Part model, mm, in its own coordinate system. A direction names the side the tool comes from. Give positions to 0.01 mm unless a question says otherwise; leave off trailing zeros. Order: outer loops, then holes, each group sorted by start corner. A loop starts at its lowest first (then second) coordinate and runs counter-clockwise, first axis right, second up. Notation, with made-up numbers: (70, 16) -> (92, 16) arc R28 ccw to (92, 43) -> close; hole circle Ø9 at (-16, 86). An arc over 180 degrees is marked (long way). Write item = value, one per line. Start each with the question number.
(1) Saw through at A-A, the plane z = -23. List the corners of the cut face in (x, y).
(2) Which spindle directions (+Z, -Z, +X, -X, +Y, -Y) get a long thin tool onto all of the face, cutting with end or side? Do faces 1 (the cylindrical face through (-23.39, 4.96, 49.78)), 2 (the cylindrical face through (-3.04, 5.8, 58.06)), 3 (the cylindrical face through (-54.248, 9.287, 0.443)). Say none if no direction does.
(3) Flat gauge pins, fed straight in: pin 1 (3.5 mm diameter, centred on y = 6, z = -59.5, fed in from +X); pin 2 (2.5 mm diameter, centred on y = 5, z = 60, fed in from -X); pin 3 (3 mm diameter, centred on x = -38.5, y = 7.5, fed in from -Z); pin 4 (3.5 mm diameter, centred on y = 5, z = -60, fed in from +X). Where does each tip first touch, or does it go through?
(4) Probe line 1 along Z through (x, y) = (-1.55, 5); line 2 along Y through (x, z) = (-1.65, -60); line 3 along Z through (x, y) = (-4, 5). List the from-to ranges inside material, lowest first. Write a range as from..to.
(5) Two-plate mould, pull along Z, no slides. Class faces 4 (the cylindrical face through (-30.35, 4.96, -57.48)), 5 (the cylindrical face through (-54.287, 0.752, 0.443)), 6 (the cylindrical face through (-45.752, 9.287, -0.396)): pulls with the +Z half, pulls with the -Z half, needs draft (parallel to the pull), parting line crosses it, or undercut.
(6) Saw through at B-B, the plane y = 5. List the corners of the cut face in (x, z), then the cut area to 3 significant figures.
(7) Saw through at C-C, the plane x = -3.5. State how many separate pieces and enclosed holes the cut face has, then the cut area to 3 significant figures.
Autodesk Inventor part; units mm, degrees
ref_plane "YZ Plane" through (0, 0, 0) normal (1, 0, 0) x (0, 1, 0)
ref_plane "XZ Plane" through (0, 0, 0) normal (0, 1, 0) x (-1, 0, 0)
ref_plane "XY Plane" through (0, 0, 0) normal (0, 0, 1) x (1, 0, 0)
sketch "Sketch1" plane through (0, 0, 0) normal (0, 1, 0) x (-1, 0, 0)
  arc A0 (0, -60) -> (0, 60) centre (0, 0) ccw construction
  arc A1 (0, -55) -> (0, 55) centre (0, 0) ccw
  arc A2 (0, -65) -> (0, 65) centre (0, 0) ccw
  line L0 (0, 65) -> (0, 55)
  line L1 (0, -55) -> (0, -65)
  line L2 (0, 65) -> (0, -65)
  line L3 (50, 41.5331) -> (50, -41.5331)
  line L4 (45, 46.9042) -> (45, -46.9042)
  line L5 (55, 34.641) -> (55, -34.641)
  point P0 (45, 31.6228)
  point P1 (45, -31.6228)
  dimension "d16" = 60
  dimension "d17" = 5
  dimension "d18" = 5
  dimension "d19" = 10
  dimension "d20" = 10
  dimension "d21" = 0
  dimension "d25" = 5
  dimension "d26" = 5
  dimension "d27" = 55
  dimension "d28" = 55
extrude "Extrusion1" add sketch "Sketch1" along normal blind 10 contours A1 L4 A2 L1 | L4 A1 L3 | A1 L3 A2 L4 | L0 A2 L4 A1 | L3 A1 | A1 L5 A2 L3 | L4 A2 L3 A1 | A1 L3 A2 L5
fillet "Fillet1" radius 10 2 edges at (-45, 5, -31.6228) (-45, 5, 31.6228)
fillet "Fillet2" radius 10 2 edges at (-55, 5, 34.641) (-55, 5, -34.641)
fillet "Fillet3" radius 2.5 16 edges at (-54.5346, 10, 34.6379) (-55, 10, 0) (-54.5346, 10, -34.6379) (-29.9649, 10, -57.681) (-29.9649, 10, 57.681) (-54.5346, 0, 34.6379) (-55, 0, 0) (-54.5346, 0, -34.6379) (-29.9649, 0, -57.681) (-29.9649, 0, 57.681) (-45, 10, 0) (-23.703, 10, -49.6303) (-23.703, 10, 49.6303) (-45, 0, 0) (-23.703, 0, -49.6303) (-23.703, 0, 49.6303)
sketch "Sketch2" plane through (0, 0, 62.5) normal (1, 0, 0) x (0, 0, -1)
  line L0 (7.5, 2.5) -> (7.5, 7.5)
  line L1 (0, 10) -> (5, 10)
  line L2 (-2.5, 2.5) -> (-2.5, 7.5)
  line L3 (0, 0) -> (5, 0)
  line L4 (120, 0) -> (125, 0)
  line L5 (127.5, 2.5) -> (127.5, 7.5)
  line L6 (120, 10) -> (125, 10)
  line L7 (117.5, 2.5) -> (117.5, 7.5)
  arc A0 (117.5, 2.5) -> (120, 0) centre (120, 2.5) ccw
  arc A1 (125, 0) -> (127.5, 2.5) centre (125, 2.5) ccw
  arc A2 (127.5, 7.5) -> (125, 10) centre (125, 7.5) ccw
  arc A3 (120, 10) -> (117.5, 7.5) centre (120, 7.5) ccw
  arc A4 (5, 0) -> (7.5, 2.5) centre (5, 2.5) ccw
  arc A5 (7.5, 7.5) -> (5, 10) centre (5, 7.5) ccw
  arc A6 (0, 10) -> (-2.5, 7.5) centre (0, 7.5) ccw
  arc A7 (-2.5, 2.5) -> (0, 0) centre (0, 2.5) ccw
  point P0 (122.5, 5)
  point P1 (2.5, 5)
hole "Hole1" at (0, 5, -60) at (0, 5, 60) direction (-1, 0, 0) diameter 4.2 depth 6
equation "\"d18\" = d17"
equation "\"d19\" = 2 * d17"
equation "\"d20\" = 2 * d17"
equation "\"d25\" = d17"
equation "\"d26\" = d17"
equation "\"d28\" = d27"
equation "\"d29\" = 2 * d17"
properties part number "Handle"
Results list:
q1.outline = (-55, 2.5) arc R2.5 ccw to (-52.5, 0) -> (-47.5, 0) arc R2.5 ccw to (-45, 2.5) -> (-45, 7.5) arc R2.5 ccw to (-47.5, 10) -> (-52.5, 10) arc R2.5 ccw to (-55, 7.5) -> close
q2.face_1 = +X, +Y, -Y
q2.face_2 = +X
q2.face_3 = +Z, -Z, -X, +Y
q3.pin_1 = 0
q3.pin_2 = -27.81
q3.pin_3 = -53.44
q3.pin_4 = -6
q4.line_1 = -64.98..-62.1, -57.9..-54.98, 54.98..57.9, 62.1..64.98
q4.line_2 = 0..2.9, 7.1..10
q4.line_3 = -64.88..-62.1, -57.9..-54.85, 54.85..57.9, 62.1..64.88
q5.face_4 = pulls with the -Z half
q5.face_5 = needs draft
q5.face_6 = undercut
q6.outline = (-55, -31.62) arc R10 ccw to (-53.18, -37.37) arc R65 ccw to (0, -65) -> (0, -62.1) -> (-6, -62.1) -> (-6, -57.9) -> (0, -57.9) -> (0, -55) arc R55 cw to (-42.78, -34.57) arc R10 cw to (-45, -28.28) -> (-45, 28.28) arc R10 cw to (-42.78, 34.57) arc R55 cw to (0, 55) -> (0, 57.9) -> (-6, 57.9) -> (-6, 62.1) -> (0, 62.1) -> (0, 65) arc R65 ccw to (-53.18, 37.37) arc R10 ccw to (-55, 31.62) -> close
q6.area = 1,800 mm^2
q7.separate_pieces = 2
q7.enclosed_holes = 2
q7.area = 162 mm^2
